The listing builds one solid part. Answer for the finished solid, in the listing's coordinates (mm). A direction names the side the tool comes from. Give positions to 0.01 mm unless a question says otherwise; leave off trailing zeros. Write each loop counter-clockwise with the first axis right and the second up, starting at its lowest first coordinate (ties: lowest second). Pieces come first, ordered by that corner, then holes. Notation, with made-up numbers: (25, 56.25) - (62, 56.25) arc R14 cw to (62, 78.25) - close; hole circle Ø11 at (13, -6.75). An arc over 180 degrees is marked (long way). Write each question's results on one line, items separated by ' | '. Start each with the question number.
Q1. Section B-B (y = 10) is taken. Determine the outline of the cut face in (x, z), plus the area to 3 significant figures.
Q2. For a pull along Z with two mould halves and no side action, classify faces 4 (the face through (-103.636, 66.599, -168.747)), 5 (the face through (-69.714, 65, 49)), 6 (the face through (46.896, 45.541, -149.93)), 7 (the face through (-3.194, 64.09, -157.185)) as pulls with the +Z half, pulls with the -Z half, needs draft (parallel to the pull), parting line crosses it, or undercut.
Q3. For faces 1 (the face through (173.3, 33.8, 103.1)), 2 (the face through (-68.728, 119.915, -17.635)), 3 (the face through (-126.53, 65.1, -74.23)), determine the directions among +Z, -Z, +X, -X, +Y, -Y from which every point of the face is accessible in a straight line to the end or side of a thin tool.
Q4. Section C-C (y = 110) is taken. Determine the outline of the cut face in (x, z).
Q5. Section A-A (z = -95) is taken. Determine the outline of the cut face in (x, y).
Q6. Flat-ended cylindrical pins translate along their axes: pin 1 Ø1 at (x, y) = (-131, 40.5) entering from +Z; pin 2 Ø4 at (x, y) = (-105, 76) entering from +Z; pin 3 Ø6 at (x, z) = (39, 129.5) entering from +Y. Find the tip coordinate at first contact, or state that the pin passes through.
Q7. Find the intervals of material crossed by probe 1 along X at (y, z) = (112, -60); probe 2 along X at (y, z) = (39.5, 91.5); probe 3 along Y at (x, z) = (173.3, -55), in increasing order.
Q8. Section D-D (z = 95) is taken. Determine the outline of the cut face in (x, y), plus the area to 3 significant figures.
```python
from build123d import *

# Parameters (mm, degrees)
BOSS_EXTRUDE2_DEPTH = 2
BOSS_EXTRUDE3_DEPTH = 128
BOSS_EXTRUDE4_DEPTH = 128
SKETCH4_R           = 21.25
SKETCH4_R_2         = 4.2
SKETCH4_R_3         = 14.25
CUT_EXTRUDE1_DEPTH  = 2
SKETCH5_R           = 10.2
CUT_EXTRUDE2_DEPTH  = 2
SKETCH6_R           = 21.25
SKETCH6_R_2         = 4.2
CUT_EXTRUDE3_DEPTH  = 2
SKETCH7_R           = 10
CUT_EXTRUDE4_DEPTH  = 2
SKETCH8_R           = 10
CUT_EXTRUDE5_DEPTH  = 2


with BuildPart() as part:
    # Sketch1 → Boss-Extrude2 (new body)
    with BuildSketch(Plane(origin=(0, 0, 0), x_dir=(1, 0, 0), z_dir=(0, 1, 0))):
        Polygon((174.285714286, -135), (174.285714286, 135), (-185.714285714, 180), (-185.714285714, -180), align=None)
    extrude(amount=BOSS_EXTRUDE2_DEPTH)



with BuildPart() as body_2:
    # Sketch2 → Boss-Extrude3 (new body)
    with BuildSketch(Plane(origin=(0, 2, 0), x_dir=(1, 0, 0), z_dir=(0, 1, 0))):
        Polygon((174.285714286, 135), (-185.714285714, 180), (-185.714285714, -180), (174.285714286, -135), align=None)
        Polygon((172.285714286, -133.234435563), (172.285714286, 133.234435563), (-183.714285714, 177.734435563), (-183.714285714, -177.734435563), align=None, mode=Mode.SUBTRACT)
    extrude(amount=BOSS_EXTRUDE3_DEPTH)


with BuildPart() as part_1:
    add(part.part)

    add(body_2.part)  # Boss-Extrude4 merges body 2
    # Sketch3 → Boss-Extrude4 (add)
    with BuildSketch(Plane(origin=(0, 2, 0), x_dir=(1, 0, 0), z_dir=(0, 1, 0))):
        Polygon((-67.714285714, 51.491616474), (-67.714285714, -165.25), (-69.714285714, -165.5), (-69.714285714, 51.491616474), (-69.714285714, 63.028269367), (-185.714285714, 81.762993886), (-185.714285714, 83.78891024), (-67.714285714, 64.731173228), align=None)
    extrude(amount=BOSS_EXTRUDE4_DEPTH)

    # Sketch4 → Cut-Extrude1 (cut)
    with BuildSketch(Plane(origin=(19.296703297, 0, 154.373626374), x_dir=(0.9922778767136677, 0, -0.12403473458920833), z_dir=(0.12403473458920831, 0, 0.9922778767136676))):
        with Locations((-151.60642933, 65)):
            Circle(SKETCH4_R)
        with Locations((-193.60642933, 65)):
            Circle(SKETCH4_R_2)
        with Locations((-109.60642933, 65)):
            Circle(SKETCH4_R_2)
        with Locations((-43.804830657, 40)):
            Circle(SKETCH4_R_3)
        with Locations((26.195169343, 40)):
            Circle(SKETCH4_R_3)
        with Locations((96.195169343, 40)):
            Circle(SKETCH4_R_3)
        with Locations((-8.804830657, 100)):
            Circle(SKETCH4_R_3)
        with Locations((61.195169343, 100)):
            Circle(SKETCH4_R_3)
    extrude(amount=-CUT_EXTRUDE1_DEPTH, mode=Mode.SUBTRACT)

    # Sketch5 → Cut-Extrude2 (cut)
    with BuildSketch(Plane(origin=(174.285714286, 0, 0), x_dir=(0, 0, -1), z_dir=(1, 0, 0))):
        with Locations((-95, 40)):
            Circle(SKETCH5_R)
        with Locations((-55, 40)):
            Circle(SKETCH5_R)
        with Locations((55, 40)):
            Circle(SKETCH5_R)
        with Locations((95, 40)):
            Circle(SKETCH5_R)
    extrude(amount=-CUT_EXTRUDE2_DEPTH, mode=Mode.SUBTRACT)

    # Sketch6 → Cut-Extrude3 (cut)
    with BuildSketch(Plane(origin=(19.296703297, 0, -154.373626374), x_dir=(-0.9922778767136676, 0, -0.12403473458920854), z_dir=(0.12403473458920855, 0, -0.9922778767136677))):
        with Locations((-72.195169343, 42)):
            Circle(SKETCH6_R)
        with Locations((-114.195169343, 42)):
            Circle(SKETCH6_R_2)
        with Locations((-30.195169343, 42)):
            Circle(SKETCH6_R_2)
        with BuildLine():
            Line((106.375385009, 43.91775074), (106.375385009, 48.66775074))
            Line((106.375385009, 48.66775074), (111.764772784, 48.66775074))
            ThreePointArc((111.764772784, 48.66775074), (124.150849168, 66.498884266), (125.575385009, 44.834745496))
            Line((125.575385009, 44.834745496), (125.575385009, 43.000755985))
            ThreePointArc((125.575385009, 43.000755985), (124.150849168, 21.336617215), (111.764772784, 39.16775074))
            Line((111.764772784, 39.16775074), (106.375385009, 39.16775074))
            Line((106.375385009, 39.16775074), (106.375385009, 43.91775074))
        make_face()
    extrude(amount=-CUT_EXTRUDE3_DEPTH, mode=Mode.SUBTRACT)

    # Sketch7 → Cut-Extrude4 (cut)
    with BuildSketch(Plane.ZY.offset(69.714285714)):
        with Locations((-16.333563693, 110)):
            Circle(SKETCH7_R)
    extrude(amount=-CUT_EXTRUDE4_DEPTH, mode=Mode.SUBTRACT)

    # Sketch8 → Cut-Extrude5 (cut)
    with BuildSketch(Plane.ZY.offset(185.714285714)):
        with Locations((-140, 40)):
            Circle(SKETCH8_R)
    extrude(amount=-CUT_EXTRUDE5_DEPTH, mode=Mode.SUBTRACT)


solid = part_1.part
```
Answers below:
1) outline: (-185.71, -180) - (174.29, -135) - (174.29, 135) - (-185.71, 180) - close; hole (-183.71, -177.73) - (172.29, -133.23) - (172.29, 133.23) - (-67.71, 163.23) - (-67.71, -64.73) - (-183.71, -83.47) - close; hole (-183.71, -81.44) - (-69.71, -63.03) - (-69.71, 163.48) - (-183.71, 177.73) - close | area: 3,380 mm2
2) face 4: undercut | face 5: undercut | face 6: parting line crosses it | face 7: pulls with the -Z half
3) face 1: +X | face 2: none | face 3: +Y
4) outline: (-185.71, -180) - (174.29, -135) - (174.29, 135) - (90.09, 145.52) - (89.84, 143.54) - (172.29, 133.23) - (172.29, -133.23) - (-183.71, -177.73) - (-183.71, -83.47) - (-67.71, -64.73) - (-67.71, -26.33) - (-69.71, -26.33) - (-69.71, -63.03) - (-183.71, -81.44) - (-183.71, 177.73) - (-69.71, 163.48) - (-69.71, -6.33) - (-67.71, -6.33) - (-67.71, 163.23) - (0.24, 154.74) - (0.49, 156.72) - (-185.71, 180) - close; (20.39, 152.22) - (69.7, 146.06) - (69.95, 148.04) - (20.63, 154.21) - close
5) outline: (-185.71, 0) - (174.29, 0) - (174.29, 29.8) - (172.29, 29.8) - (172.29, 2) - (-183.71, 2) - (-183.71, 130) - (-185.71, 130) - close; (172.29, 50.2) - (174.29, 50.2) - (174.29, 130) - (172.29, 130) - close
6) pin 1: stops at z = 173.22 | pin 2: stops at z = 170.16 | pin 3: stops at y = 2
7) probe 1: x = -185.71 to -183.71, -69.71 to -67.71, 172.29 to 174.29 | probe 2: x = -185.71 to -183.71, -69.71 to -67.71 | probe 3: y = 0 to 29.8, 50.2 to 130
8) outline: (-185.71, 0) - (174.29, 0) - (174.29, 29.8) - (172.29, 29.8) - (172.29, 2) - (-67.71, 2) - (-67.71, 130) - (-69.71, 130) - (-69.71, 2) - (-183.71, 2) - (-183.71, 130) - (-185.71, 130) - close; (172.29, 50.2) - (174.29, 50.2) - (174.29, 130) - (172.29, 130) - close | area: 1,450 mm2
